```python
from build123d import *

# Parameters (mm, degrees)
SKETCH_W        = 130
SKETCH_H        = 90
PAD_DEPTH       = 387.5
POCKET_DEPTH    = 36.5
SKETCH002_R     = 19
POCKET001_DEPTH = 90.001
SKETCH003_W     = 79
SKETCH003_H     = 79
POCKET002_DEPTH = 13


with BuildPart() as part:
    # Sketch → Pad (new body, symmetric)
    with BuildSketch(Plane.XY):
        Rectangle(SKETCH_W, SKETCH_H)
    extrude(amount=PAD_DEPTH, both=True)

    # Sketch001 → Pocket (cut)
    with BuildSketch(Plane.XZ.offset(45)):
        Polygon((0, 172.5), (-31.75, 172.5), (-31.75, 72.5), (-22.5, 72.5), (-22.5, -322.5), (0, -322.5), align=None)
    pocket = extrude(amount=-POCKET_DEPTH, mode=Mode.SUBTRACT)

    # Mirrored: Pocket across Sketch001 V_Axis
    add(pocket.mirror(Plane(origin=(0, -45, 0), x_dir=(0, -1, 0), z_dir=(1, 0, 0))), mode=Mode.SUBTRACT)

    # Sketch002 → Pocket001 (cut, through all)
    with BuildSketch(Plane.XZ.offset(45)):
        with Locations((0, 226.5)):
            Circle(SKETCH002_R)
    extrude(amount=-POCKET001_DEPTH, mode=Mode.SUBTRACT)

    # Sketch003 → Pocket002 (cut)
    with BuildSketch(Plane.XZ.offset(45)):
        with Locations((0, 229.74)):
            Rectangle(SKETCH003_W, SKETCH003_H)
    extrude(amount=-POCKET002_DEPTH, mode=Mode.SUBTRACT)


solid = part.part
```
Input: part model. Units: mm. Frame: model coordinates. A direction names the side the tool comes from. Round coordinates to 2 decimals unless told otherwise and drop trailing zeros. Loops run counter-clockwise (first coordinate to the right, second up) from the corner with the lowest first, then second, coordinate; pieces in that order, holes last. Notation, with made-up numbers: M 41.25,77.5 L 93.25,77.5 A31 cw 93.25,104.5 Z; hole C -21,64 d11. An arc over 180 degrees is marked long. Answer in a Markdown table with one row per item. Add a question column.
1. Ray query, probe 1 along Z at (x, y) = (0, -16); probe 2 along Z at (x, y) = (0, 27); probe 3 along X at (y, z) = (26, 226). Return the intervals inside material, ascending.
2. Section C-C (y = -23). Output: boundary loops of the cut face in (x, z), and give its area (3 significant figures).
3. Section B-B (z = 226.5). Output: boundary loops of the cut face in (x, y).
4. Section D-D (z = 140). Output: boundary loops of the cut face in (x, y).
5. Mould query, pull axis Z, two halves, no side actions, for faces 3 (the face through (-22.5, -27, -122)), 4 (the face through (-1, -39, 190.24)), 5 (the face through (65, -1, 5)), 6 (the face through (-1, 1, -387.5)). Classes: released by +Z, released by -Z, zero draft, split by the parting line, or undercut.
6. Section A-A (x = 0). Output: boundary loops of the cut face in (y, z), and give its area (3 significant figures).
7. Set-up query: faces 1 (the face through (-30, -45, 5)), 2 (the face through (-1, -32, 248)). Return all of +Z, -Z, +X, -X, +Y, -Y with unobstructed straight access to the full face (end or side cutting, diameter ignored); none if empty.
Values follow:
| question | item | result |
|---|---|---|
| 1 | probe 1 | -387.5 to -322.5, 172.5 to 207.5, 245.5 to 387.5 |
| 1 | probe 2 | -387.5 to 207.5, 245.5 to 387.5 |
| 1 | probe 3 | -65 to -18.99, 18.99 to 65 |
| 2 | outline | M -65,-387.5 L 65,-387.5 L 65,387.5 L -65,387.5 Z; hole M -31.75,72.5 L -22.5,72.5 L -22.5,-322.5 L 22.5,-322.5 L 22.5,72.5 L 31.75,72.5 L 31.75,172.5 L -31.75,172.5 Z; hole C 0,226.5 d38 |
| 2 | area | 75,500 mm^2 |
| 3 | outline | M -65,-45 L -39.5,-45 L -39.5,-32 L -19,-32 L -19,45 L -65,45 Z; M 19,-32 L 39.5,-32 L 39.5,-45 L 65,-45 L 65,45 L 19,45 Z |
| 4 | outline | M -65,-45 L -31.75,-45 L -31.75,-8.5 L 31.75,-8.5 L 31.75,-45 L 65,-45 L 65,45 L -65,45 Z |
| 5 | face 3 | undercut |
| 5 | face 4 | undercut |
| 5 | face 5 | zero draft |
| 5 | face 6 | released by -Z |
| 6 | outline | M -45,-387.5 L 45,-387.5 L 45,207.5 L -32,207.5 L -32,190.24 L -45,190.24 L -45,172.5 L -8.5,172.5 L -8.5,-322.5 L -45,-322.5 Z; M -45,269.24 L -32,269.24 L -32,245.5 L 45,245.5 L 45,387.5 L -45,387.5 Z |
| 6 | area | 47,700 mm^2 |
| 7 | face 1 | +Z, -Z, +X, -X, -Y |
| 7 | face 2 | -Y |
